CAD build for the part. Positions are in the model's coordinates, mm. A direction names the side the tool comes from. Coordinates: 2 decimals unless noted, no trailing zeros. Order: outer loops, then holes, each group sorted by start corner. A loop starts at its lowest first (then second) coordinate and runs counter-clockwise, first axis right, second up. Notation, with made-up numbers: M 87.5,89 L 110.5,89 A28 cw 110.5,125 Z; hole C 85.25,33.5 d5. An arc over 180 degrees is marked long. Write item = value, one per line.
from build123d import *

# Parameters (mm, degrees)
EXTRUDE_1_DEPTH     = 5
SKETCH_2_W          = 5
SKETCH_2_H          = 42
EXTRUDE_2_DEPTH     = 66
SKETCH_3_R          = 11.5
SKETCH_3_R_2        = 1.5
CUT_EXTRUDE_1_DEPTH = 5
SKETCH_5_R          = 2
SKETCH_5_R_2        = 2.75
CUT_EXTRUDE_2_DEPTH = 80.818544211
FILLET_1_R          = 10
FILLET_2_R          = 10


with BuildPart() as part:
    # 草图1 → 凸台-拉伸1 (new body)
    with BuildSketch(Plane.XY):
        with BuildLine():
            Line((13.564659966, -21), (25, -21))
            Line((25, -21), (25, 21))
            Line((25, 21), (13.564659966, 21))
            ThreePointArc((13.564659966, 21), (0, 25), (-13.564659966, 21))
            Line((-13.564659966, 21), (-40, 21))
            Line((-40, 21), (-40, -21))
            Line((-40, -21), (-13.564659966, -21))
            ThreePointArc((-13.564659966, -21), (0, -25), (13.564659966, -21))
        make_face()
    extrude(amount=EXTRUDE_1_DEPTH)

    # 草图2 → 凸台-拉伸2 (add)
    with BuildSketch(Plane.XY.offset(5)):
        with Locations((-42.5, 0)):
            Rectangle(SKETCH_2_W, SKETCH_2_H)
    extrude(amount=-EXTRUDE_2_DEPTH)

    # 草图3 → 切除-拉伸1 (cut)
    with BuildSketch(Plane.ZY.offset(45)):
        with Locations((-40, 0)):
            Circle(SKETCH_3_R)
        with Locations((-55.5, 15.5)):
            Circle(SKETCH_3_R_2)
        with Locations((-55.5, -15.5)):
            Circle(SKETCH_3_R_2)
        with Locations((-24.5, 15.5)):
            Circle(SKETCH_3_R_2)
        with Locations((-24.5, -15.5)):
            Circle(SKETCH_3_R_2)
        with Locations((34.5, 74.5)):
            Circle(SKETCH_3_R_2)
    extrude(amount=-CUT_EXTRUDE_1_DEPTH, mode=Mode.SUBTRACT)

    # 草图5 → 切除-拉伸2 (cut, through all)
    with BuildSketch(Plane(origin=(0, 0, 0), x_dir=(-1, 0, 0), z_dir=(0, 0, -1))):
        with Locations((0, 8)):
            Circle(SKETCH_5_R)
        with Locations((8, 0)):
            Circle(SKETCH_5_R)
        with Locations((0, -8)):
            Circle(SKETCH_5_R)
        with Locations((-8, 0)):
            Circle(SKETCH_5_R)
        Circle(SKETCH_5_R_2)
    extrude(amount=-CUT_EXTRUDE_2_DEPTH, mode=Mode.SUBTRACT)

    # 圆角1
    fillet_1_edges = [part.edges().sort_by_distance(p)[0] for p in [
        (-40, 0, 0),
    ]]
    fillet(fillet_1_edges, radius=FILLET_1_R)

    # 圆角2
    fillet_2_edges = [part.edges().sort_by_distance(p)[0] for p in [
        (25, -21, 2.5),
        (25, 21, 2.5),
        (-42.5, 21, -61),
        (-42.5, -21, -61),
    ]]
    fillet(fillet_2_edges, radius=FILLET_2_R)


solid = part.part
(1) Wall check: line 1 (Y direction, x = 0, z = 2); line 2 (Y direction, x = -42.85, z = -24.5); line 3 (Y direction, x = -41.25, z = -40). Give the ranges that are in metal, low to high. Write a range as from..to.
Evaluation:
line_1 = -25..-10, -6..-2.75, 2.75..6, 10..25
line_2 = -21..-17, -14..14, 17..21
line_3 = -21..-11.5, 11.5..21
(2) Slice it at C-C, the plane y = -15.5. Write the cut outline in (x, z), then the cut area to 3 significant figures.
Evaluation:
outline = M -45,-59.93 L -40,-59.93 L -40,-57 L -45,-57 Z; M -45,-54 L -40,-54 L -40,-26 L -45,-26 Z; M -45,-23 L -40,-23 L -40,-10 A10 cw -30,0 L 23.93,0 L 23.93,5 L -45,5 Z
area = 636 mm²
(3) Slice it at B-B, the plane x = 8. Write the cut outline in (y, z), then the cut area to 3 significant figures.
Evaluation:
outline = M -23.69,0 L -2,0 L -2,5 L -23.69,5 Z; M 2,0 L 23.69,0 L 23.69,5 L 2,5 Z
area = 217 mm²
(4) Slice it at A-A, the plane z = -40. Write the cut outline in (x, y).
Evaluation:
outline = M -45,-21 L -40,-21 L -40,-11.5 L -45,-11.5 Z; M -45,11.5 L -40,11.5 L -40,21 L -45,21 Z
(5) Pull direction X, two halves, no side cores. Call faces 1 (the face through (-3, 0, 0)), 2 (the face through (-6, 0, 2)), 3 (the face through (-37.15, -0.29, -3.01)): +X half, -X half, draft (parallel to the pull), parting line (faces both ways), or undercut.
Evaluation:
face_1 = draft
face_2 = undercut
face_3 = +X half
(6) Slice it at D-D, the plane z = -55.5. Write the cut outline in (x, y), then the cut area to 3 significant figures.
Evaluation:
outline = M -45,-19.93 L -40,-19.93 L -40,-17 L -45,-17 Z; M -45,-14 L -40,-14 L -40,14 L -45,14 Z; M -45,17 L -40,17 L -40,19.93 L -45,19.93 Z
area = 169 mm²
(7) Tool access for faces 4 (the face through (-40, -5, -29)), 5 (the face through (-42.46, -18.15, -57.99)), 6 (the face through (-41, -21, -15)), 7 (the face through (-41, 21, -15)), 8 (the face through (-42.54, 15.95, -54.07)): list every direction of +Z, -Z, +X, -X, +Y, -Y with a clear straight run to the whole face (end or side of a thin tool).
Evaluation:
face_4 = -Z, +X, +Y, -Y
face_5 = -Z, +X, -X, -Y
face_6 = +Z, -Z, -X, -Y
face_7 = +Z, -Z, -X, +Y
face_8 = +X, -X
(8) Pin check, flat tips, straight feed: pin 1 Ø8 at (x, y) = (9, -15) entering from -Z; pin 2 Ø21 at (y, z) = (4, -29) entering from +X. Stop position of each tip, or through.
Evaluation:
pin_1 = 0
pin_2 = -40
